from build123d import *

# Parameters (mm, degrees)
P01_STANDOFF_START             = 14.3
SK_P01_STANDOFF_R              = 2
P01_STANDOFF_DEPTH             = 8
P02_STANDOFF_START             = 14.3
SK_P02_STANDOFF_R              = 2
P02_STANDOFF_DEPTH             = 8
P03_STANDOFF_START             = 14.3
SK_P03_STANDOFF_R              = 2
P03_STANDOFF_DEPTH             = 8
P04_STANDOFF_START             = 14.3
SK_P04_STANDOFF_R              = 2
P04_STANDOFF_DEPTH             = 8
P05_CARRIERBOARD_START         = 12.7
SK_P05_CARRIERBOARD_W          = 60
SK_P05_CARRIERBOARD_H          = 40
P05_CARRIERBOARD_DEPTH         = 1.6
P06_INA2603SENSOR_START        = 10
SK_P06_INA2603SENSOR_W         = 22.9
SK_P06_INA2603SENSOR_H         = 23
P06_INA2603SENSOR_DEPTH        = 2.7
SK_P07_INA260TERMINALBLOCK_W   = 10
SK_P07_INA260TERMINALBLOCK_H   = 8
P07_INA260TERMINALBLOCK_DEPTH  = 10
P08_BUCKBD36V50F55V_START      = 3.2
SK_P08_BUCKBD36V50F55V_W       = 25.4
SK_P08_BUCKBD36V50F55V_H       = 25.4
P08_BUCKBD36V50F55V_DEPTH      = 9.5
P09_JSTXHHEADERSFACEDOWN_START = 2.3
SK_P09_JSTXHHEADERSFACEDOWN_W  = 56
SK_P09_JSTXHHEADERSFACEDOWN_H  = 8
P09_JSTXHHEADERSFACEDOWN_DEPTH = 10.4


with BuildPart() as part:
    # SK_P01_Standoff → P01_Standoff (new body)
    with BuildSketch(Plane(origin=(0, 0, 0), x_dir=(1, 0, 0), z_dir=(0, 1, 0)).offset(P01_STANDOFF_START)):
        with Locations(Location((-26, 18, 0), (0, 0, 270))):
            Circle(SK_P01_STANDOFF_R)
    extrude(amount=P01_STANDOFF_DEPTH)



with BuildPart() as body_2:
    # SK_P02_Standoff → P02_Standoff (new body)
    with BuildSketch(Plane(origin=(0, 0, 0), x_dir=(1, 0, 0), z_dir=(0, 1, 0)).offset(P02_STANDOFF_START)):
        with Locations(Location((-26, -16, 0), (0, 0, 270))):
            Circle(SK_P02_STANDOFF_R)
    extrude(amount=P02_STANDOFF_DEPTH)


with BuildPart() as body_3:
    # SK_P03_Standoff → P03_Standoff (new body)
    with BuildSketch(Plane(origin=(0, 0, 0), x_dir=(1, 0, 0), z_dir=(0, 1, 0)).offset(P03_STANDOFF_START)):
        with Locations(Location((26, 18, 0), (0, 0, 270))):
            Circle(SK_P03_STANDOFF_R)
    extrude(amount=P03_STANDOFF_DEPTH)


with BuildPart() as body_4:
    # SK_P04_Standoff → P04_Standoff (new body)
    with BuildSketch(Plane(origin=(0, 0, 0), x_dir=(1, 0, 0), z_dir=(0, 1, 0)).offset(P04_STANDOFF_START)):
        with Locations(Location((26, -16, 0), (0, 0, 270))):
            Circle(SK_P04_STANDOFF_R)
    extrude(amount=P04_STANDOFF_DEPTH)


with BuildPart() as part_1:
    add(part.part)

    add(body_2.part)  # P05_Carrierboard merges body 2

    add(body_3.part)  # P05_Carrierboard merges body 3

    add(body_4.part)  # P05_Carrierboard merges body 4
    # SK_P05_Carrierboard → P05_Carrierboard (add)
    with BuildSketch(Plane(origin=(0, 0, 0), x_dir=(1, 0, 0), z_dir=(0, 1, 0)).offset(P05_CARRIERBOARD_START)):
        Rectangle(SK_P05_CARRIERBOARD_W, SK_P05_CARRIERBOARD_H)
    extrude(amount=P05_CARRIERBOARD_DEPTH)

    # SK_P06_INA2603sensor → P06_INA2603sensor (add)
    with BuildSketch(Plane(origin=(0, 0, 0), x_dir=(1, 0, 0), z_dir=(0, 1, 0)).offset(P06_INA2603SENSOR_START)):
        with Locations((-16.55, 4.5)):
            Rectangle(SK_P06_INA2603SENSOR_W, SK_P06_INA2603SENSOR_H)
    extrude(amount=P06_INA2603SENSOR_DEPTH)

    # SK_P07_INA260terminalblock → P07_INA260terminalblock (add)
    with BuildSketch(Plane(origin=(0, 0, 0), x_dir=(1, 0, 0), z_dir=(0, 1, 0))):
        with Locations((-20, 10)):
            Rectangle(SK_P07_INA260TERMINALBLOCK_W, SK_P07_INA260TERMINALBLOCK_H)
    extrude(amount=P07_INA260TERMINALBLOCK_DEPTH)

    # SK_P08_BuckBD36V50F55V → P08_BuckBD36V50F55V (add)
    with BuildSketch(Plane(origin=(0, 0, 0), x_dir=(1, 0, 0), z_dir=(0, 1, 0)).offset(P08_BUCKBD36V50F55V_START)):
        with Locations((14.3, 3.3)):
            Rectangle(SK_P08_BUCKBD36V50F55V_W, SK_P08_BUCKBD36V50F55V_H)
    extrude(amount=P08_BUCKBD36V50F55V_DEPTH)

    # SK_P09_JSTXHheadersfacedown → P09_JSTXHheadersfacedown (add)
    with BuildSketch(Plane(origin=(0, 0, 0), x_dir=(1, 0, 0), z_dir=(0, 1, 0)).offset(P09_JSTXHHEADERSFACEDOWN_START)):
        with Locations((0, -15)):
            Rectangle(SK_P09_JSTXHHEADERSFACEDOWN_W, SK_P09_JSTXHHEADERSFACEDOWN_H)
    extrude(amount=P09_JSTXHHEADERSFACEDOWN_DEPTH)


solid = part_1.part
Can you work these out from the model? Positions are in its coordinate system, mm. A direction names the side the tool comes from. Round coordinates to 2 decimals unless told otherwise and drop trailing zeros. Loops run counter-clockwise (first coordinate to the right, second up) from the corner with the lowest first, then second, coordinate; pieces in that order, holes last. Notation, with made-up numbers: (64, -33) - (119, -33) arc R27 cw to (119, -7) - close; hole circle Ø8 at (13.5, 45). An arc over 180 degrees is marked (long way). Use CSV: the item, a comma, the result in double quotes. Start each with the question number.
1) For pin 1 Ø5 at (x, y) = (-2.5, 18) entering from -Z; pin 2 Ø12 at (y, z) = (16, -2) entering from -X; pin 3 Ø6.5 at (x, z) = (9, 17) entering from -Y; pin 4 Ø2 at (y, z) = (11, -5.5) entering from -X, each with a flat end and sliding along its axis, tell me the tip position at first contact or that it passes through.
2) Please list where these lines run through material, in increasing order: probe 1 along X at (y, z) = (11, -4.5); probe 2 along X at (y, z) = (5, -13.5); probe 3 along Z at (x, y) = (14.5, 5.5). Write a range as [from, to].
3) If we section it at C-C on y = 18: Write out the boundary of the cut face in (x, z).
4) If we section it at A-A on z = 2: Write out the boundary of the cut face in (x, y).
5) We'd pull the mould along X, two halves only. Please class faces 5 (the flat face through (-20, 5, -14)), 6 (the flat face through (0, 14.3, 0)), 7 (the flat face through (-28, 7, 15)): released by +X, released by -X, zero draft, split by the parting line, or undercut.
6) If we section it at B-B on x = -22: Write out the boundary of the cut face in (y, z).
7) For faces 1 (the flat face through (-20, 5, -6)), 2 (the flat face through (27, 8, -3)), 3 (the flat face through (1.6, 8, -3)), 4 (the flat face through (-17, 11, -16)), which set-ups out of +Z, -Z, +X, -X, +Y, -Y let a thin tool reach every point of the face, with its end or its side?
8) If we section it at D-D on z = 16: Write out the boundary of the cut face in (x, y).
Geometry results:
1,pin 1,"passes through"
1,pin 2,"stops at x = -30"
1,pin 3,"stops at y = 2.3"
1,pin 4,"stops at x = -28"
2,probe 1,"x = [-28, -5.1], [1.6, 27]"
2,probe 2,"x = [-25, -15], [1.6, 27]"
2,probe 3,"z = [-16, 9.4], [11, 19]"
3,outline,"circle Ø4 at (-26, -18); circle Ø4 at (-26, 16); circle Ø4 at (26, -18); circle Ø4 at (26, 16)"
4,outline,"(-30, 12.7) - (-28, 12.7) - (-28, 10) - (-5.1, 10) - (-5.1, 12.7) - (1.6, 12.7) - (1.6, 3.2) - (27, 3.2) - (27, 12.7) - (30, 12.7) - (30, 14.3) - (-30, 14.3) - close"
5,face 5,"zero draft"
5,face 6,"undercut"
5,face 7,"released by -X"
6,outline,"(0, -14) - (10, -14) - (10, -16) - (12.7, -16) - (12.7, -20) - (14.3, -20) - (14.3, 20) - (12.7, 20) - (12.7, 19) - (2.3, 19) - (2.3, 11) - (12.7, 11) - (12.7, 7) - (10, 7) - (10, -6) - (0, -6) - close"
7,face 1,"-X, -Y"
7,face 2,"-Z, +X, -Y"
7,face 3,"-Z, -Y"
7,face 4,"-Z, +X, -X, -Y"
8,outline,"(-30, 12.7) - (-28, 12.7) - (-28, 2.3) - (28, 2.3) - (28, 12.7) - (30, 12.7) - (30, 14.3) - (28, 14.3) - (28, 22.3) - (24, 22.3) - (24, 14.3) - (-24, 14.3) - (-24, 22.3) - (-28, 22.3) - (-28, 14.3) - (-30, 14.3) - close"
